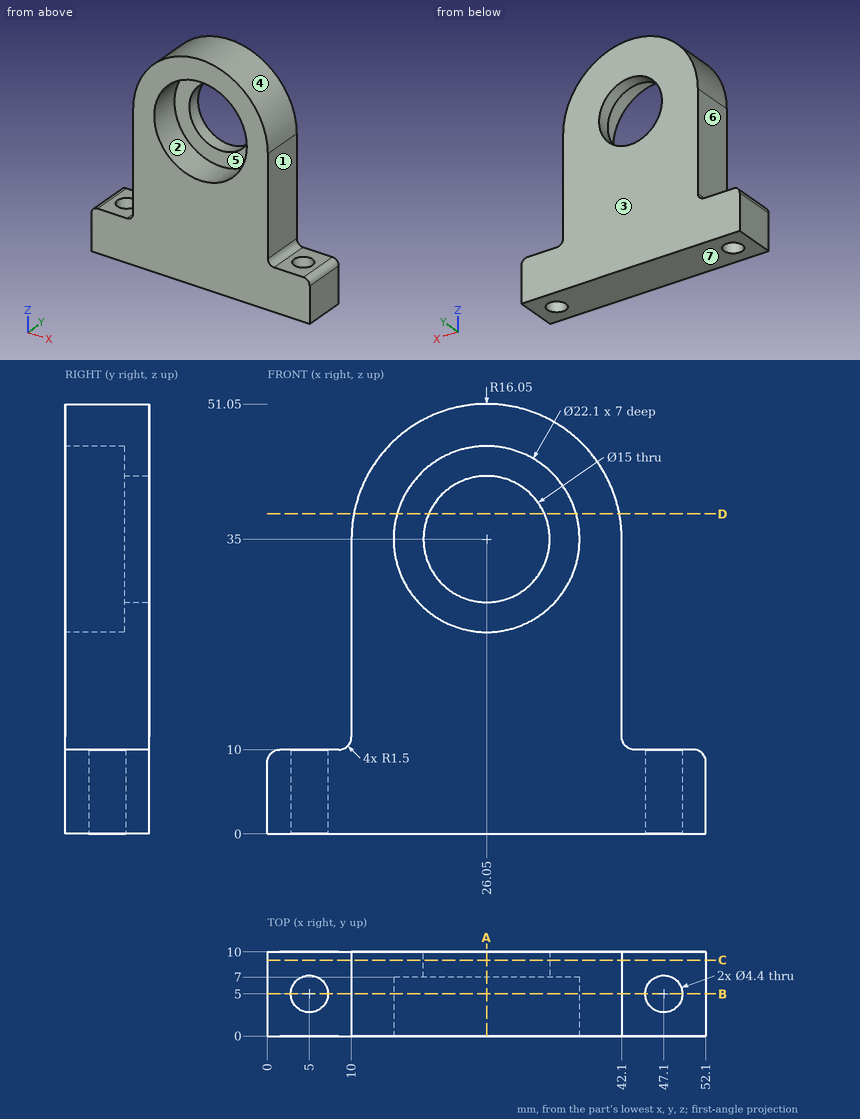
Geometry: see drawing. Coordinates: mm, zero at the bounding-box minimum. A direction names the side the tool comes from. Give positions to 0.01 mm unless a question says otherwise; leave off trailing zeros. Write each loop counter-clockwise with the first axis right and the second up, starting at its lowest first coordinate (ties: lowest second). Pieces come first, ordered by that corner, then holes. Notation, with made-up numbers: M 10,75.5 L 50,75.5 A12 ccw 50,81.5 Z; hole C 48,69.25 d3. An arc over 180 degrees is marked long. Answer in a Markdown table with one row per item. Add a question column.
(1) First-contact query: pin 1 (5 mm diameter, centred on y = 5, z = 20, fed in from +X); pin 2 (6 mm diameter, centred on x = 36.5, y = 4.5, fed in from +Z); pin 3 (1 mm diameter, centred on x = 12.5, y = 2.5, fed in from +Z). Flat tips, straight axial feed; report the tip coordinate or a pass-through.
(2) Reachability of the marked faces 1, 2 and 3 from +Z, -Z, +X, -X, +Y, -Y: full face, straight path, thin tool, end or side. Return the list, or none.
(3) Section C-C on y = 9. Return loops of the section in (x, z), and give its area (3 significant figures).
(4) Section B-B on y = 5. Return loops of the section in (x, z), and give its area (3 significant figures).
(5) Ray query, line 1 (Y direction, x = 5, z = 2); line 2 (X direction, y = 6.75, z = 15.5); line 3 (X direction, y = 4.5, z = 43). Return the intervals inside material, ascending.
(6) Section A-A on x = 26.05. Return loops of the section in (y, z), and give its area (3 significant figures).
(7) Section D-D on z = 38. Return loops of the section in (x, y).
(8) Mould query, pull axis Z, two halves, no side actions, for the marked faces 4, 5, 6 and 7. Classes: +Z half, -Z half, draft (parallel to the pull), parting line (faces both ways), or undercut.
Result set:
| question | item | result |
|---|---|---|
| 1 | pin 1 | stops at x = 42.1 |
| 1 | pin 2 | stops at z = 49.22 |
| 1 | pin 3 | stops at z = 44.34 |
| 2 | face 1 | +Z, +X, +Y, -Y |
| 2 | face 2 | -Y |
| 2 | face 3 | +Z, -Z, +X, -X, +Y |
| 3 | outline | M 0,0 L 52.1,0 L 52.1,8.5 A1.5 ccw 50.6,10 L 43.6,10 A1.5 cw 42.1,11.5 L 42.1,35 A16.05 ccw 10,35 L 10,11.5 A1.5 cw 8.5,10 L 1.5,10 A1.5 ccw 0,8.5 Z; hole C 26.05,35 d15 |
| 3 | area | 1,550 mm^2 |
| 4 | outline | M 0,0 L 2.8,0 L 2.8,10 L 1.5,10 A1.5 ccw 0,8.5 Z; M 7.2,0 L 44.9,0 L 44.9,10 L 43.6,10 A1.5 cw 42.1,11.5 L 42.1,35 A16.05 ccw 10,35 L 10,11.5 A1.5 cw 8.5,10 L 7.2,10 Z; M 49.3,0 L 52.1,0 L 52.1,8.5 A1.5 ccw 50.6,10 L 49.3,10 Z; hole C 26.05,35 d22.1 |
| 4 | area | 1,260 mm^2 |
| 5 | line 1 | y = 0 to 2.8, 7.2 to 10 |
| 5 | line 2 | x = 10 to 42.1 |
| 5 | line 3 | x = 12.14 to 18.43, 33.67 to 39.96 |
| 6 | outline | M 0,0 L 10,0 L 10,27.5 L 7,27.5 L 7,23.95 L 0,23.95 Z; M 0,46.05 L 7,46.05 L 7,42.5 L 10,42.5 L 10,51.05 L 0,51.05 Z |
| 6 | area | 311 mm^2 |
| 7 | outline | M 10.28,0 L 15.42,0 L 15.42,7 L 19.18,7 L 19.18,10 L 10.28,10 Z; M 32.92,7 L 36.68,7 L 36.68,0 L 41.82,0 L 41.82,10 L 32.92,10 Z |
| 8 | face 4 | +Z half |
| 8 | face 5 | undercut |
| 8 | face 6 | draft |
| 8 | face 7 | -Z half |
